Source: CAD feature listing. Evaluate the final solid. Frame: model axes, mm. Give positions to 0.01 mm unless a question says otherwise; leave off trailing zeros. Loops run counter-clockwise (first coordinate to the right, second up) from the corner with the lowest first, then second, coordinate; pieces in that order, holes last. Notation, with made-up numbers: (71.25, -17.75) - (102.25, -17.75) arc R28 ccw to (102.25, 16.25) - close; hole circle Ø3 at (21, 65.25). An arc over 180 degrees is marked (long way). Write each question's results on one line, items separated by ' | '. Start each with the question number.
(1) Cut plane C-C on x = -52. Return the cut outline in (y, z), then the cut area to 3 significant figures.
(2) Cut plane A-A on x = 0. Return the cut outline in (y, z), then the cut area to 3 significant figures.
(3) Cut plane D-D on y = -70.5. Return the cut outline in (x, z).
(4) Material intervals for line 1 along Z through (x, y) = (218, 0); line 2 along X through (y, z) = (-1.5, 68); line 3 along X through (y, z) = (90.5, 51), sorted ascending. Write a range as [from, to].
(5) Pull-direction query (X, two-part tool) for faces 1 (the flat face through (168, 137, 101.6)), 2 (the cylindrical face through (-228.38, 10.05, 50.09)), 3 (the cylindrical face through (0.8, -222.1, 57.1)); classes: pulls with the +X half, pulls with the -X half, needs draft (parallel to the pull), parting line crosses it, or undercut.
(6) Contact query for flat-ended pins moving along their axis: pin 1 (11.5 mm diameter, centred on x = 0, z = 50.8, fed in from +Y); pin 2 (1 mm diameter, centred on y = -92, z = 27.5, fed in from +X); pin 3 (10 mm diameter, centred on x = 178, z = 51, fed in from -Y); pin 4 (2 mm diameter, centred on y = 149.5, z = 62.5, fed in from +X). Output: stop coordinate, or through.
from build123d import *

# Parameters (mm, degrees)
SKETCH1_R           = 228.6
BOSS_EXTRUDE1_DEPTH = 101.6
SKETCH2_R           = 215.9
CUT_EXTRUDE1_DEPTH  = 102.6
SKETCH3_R           = 6.35
CUT_EXTRUDE2_DEPTH  = 458.2
SKETCH4_R           = 6.35
CUT_EXTRUDE3_DEPTH  = 458.2000001


with BuildPart() as part:
    # Sketch1 → Boss-Extrude1 (new body)
    with BuildSketch(Plane.XY):
        Circle(SKETCH1_R)
    extrude(amount=BOSS_EXTRUDE1_DEPTH)

    # Sketch2 → Cut-Extrude1 (cut, through all)
    with BuildSketch(Plane.XY.offset(101.6)):
        Circle(SKETCH2_R)
    extrude(amount=-CUT_EXTRUDE1_DEPTH, mode=Mode.SUBTRACT)

    # Sketch3 → Cut-Extrude2 (cut, through all)
    with BuildSketch(Plane(origin=(0, 228.6, 0), x_dir=(-1, 0, 0), z_dir=(0, 1, 0))):
        with Locations((0, 50.8)):
            Circle(SKETCH3_R)
    extrude(amount=-CUT_EXTRUDE2_DEPTH, mode=Mode.SUBTRACT)

    # Sketch4 → Cut-Extrude3 (cut, through all)
    with BuildSketch(Plane(origin=(228.6, 0, 0), x_dir=(0, 0, -1), z_dir=(1, 0, 0))):
        with Locations((-50.8, 0)):
            Circle(SKETCH4_R)
    extrude(amount=-CUT_EXTRUDE3_DEPTH, mode=Mode.SUBTRACT)


solid = part.part
Ans:
1) outline: (-222.61, 0) - (-209.54, 0) - (-209.54, 101.6) - (-222.61, 101.6) - close; (209.54, 0) - (222.61, 0) - (222.61, 101.6) - (209.54, 101.6) - close | area: 2,650 mm^2
2) outline: (-228.6, 0) - (-215.9, 0) - (-215.9, 44.45) - (-228.6, 44.45) - close; (-228.6, 57.15) - (-215.9, 57.15) - (-215.9, 101.6) - (-228.6, 101.6) - close; (215.9, 0) - (228.6, 0) - (228.6, 44.45) - (215.9, 44.45) - close; (215.9, 57.15) - (228.6, 57.15) - (228.6, 101.6) - (215.9, 101.6) - close | area: 2,260 mm^2
3) outline: (-217.46, 0) - (-204.07, 0) - (-204.07, 101.6) - (-217.46, 101.6) - close; (204.07, 0) - (217.46, 0) - (217.46, 101.6) - (204.07, 101.6) - close
4) line 1: [0, 44.45], [57.15, 101.6] | line 2: [-228.6, -215.89], [215.89, 228.6] | line 3: [-209.92, -196.02], [196.02, 209.92]
5) face 1: needs draft | face 2: parting line crosses it | face 3: undercut
6) pin 1: through | pin 2: x = 209.49 | pin 3: y = -149.43 | pin 4: x = 173.8
